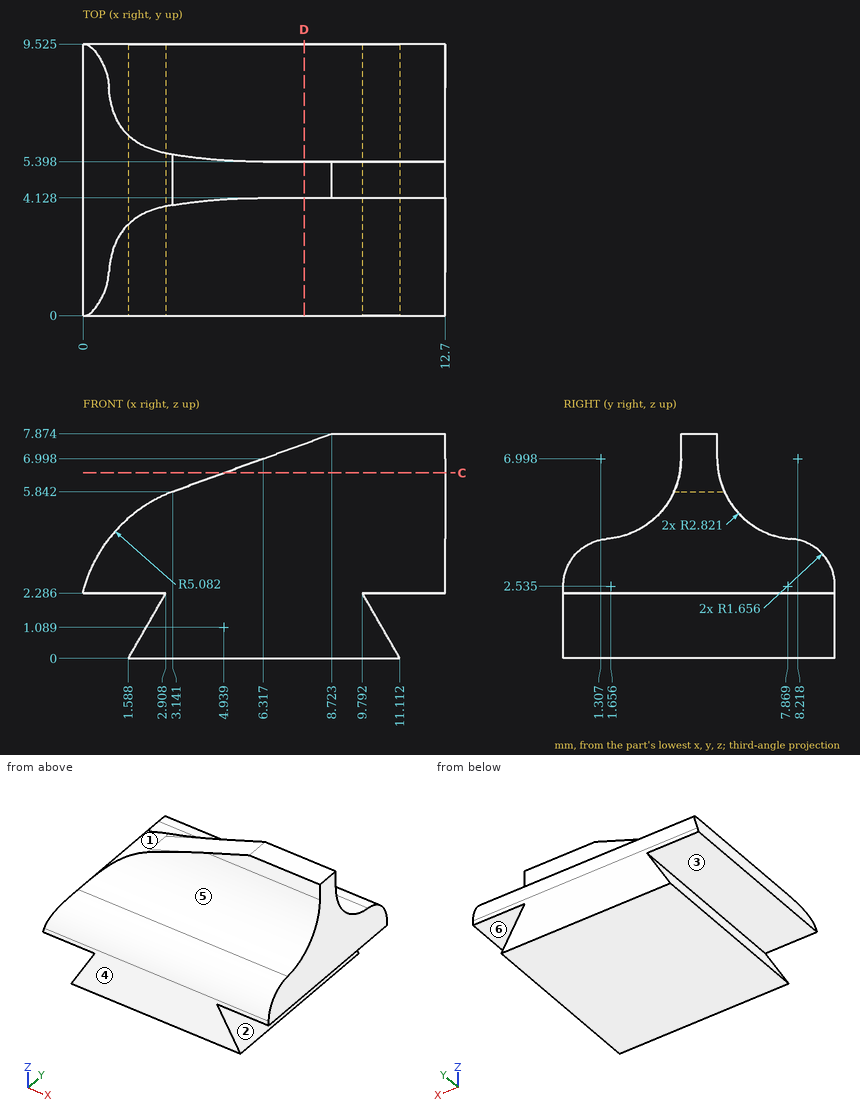
Input: dimensioned drawing with shaded views. Units: mm. Origin: part minimum x, y, z. A direction names the side the tool comes from. Give positions to 0.01 mm unless a question says otherwise; leave off trailing zeros. Loops run counter-clockwise (first coordinate to the right, second up) from the corner with the lowest first, then second, coordinate; pieces in that order, holes last. Notation, with made-up numbers: (46.5, 41) -> (103.5, 41) arc R18 ccw to (103.5, 52) -> close; hole circle Ø11 at (-31.5, -18). An arc over 180 degrees is marked (long way). Return JSON: item names as keys, results as strings.
Item 1: Mould query, pull axis Z, two halves, no side actions, for the marked faces 4, 5 and 6. Classes: released by +Z, released by -Z, zero draft, split by the parting line, or undercut.
Filled in:
{"face 4": "zero draft", "face 5": "released by +Z", "face 6": "undercut"}
Item 2: Pin query (flat end, axial travel): P1, Ø0.9, axis at x = 11, y = 6, coming from the -Z side; P2, Ø1.5, axis at x = 7, y = 1.5, coming from the +Z side; P3, Ø1.5, axis at x = 2.5, y = 5, coming from the +Z side. Return the tip coordinate at first contact, or that it passes through.
Filled in:
{"P1": "z = 0", "P2": "z = 4.34", "P3": "z = 5.88"}
Item 3: Access query for the marked faces 1, 2 and 3. Directions: +Z, -Z, +X, -X, +Y, -Y. A direction counts if a zero-diameter tool reaches every point of the face in a straight line with its end or side. Return the directions, or none.
Filled in:
{"face 1": "+Z, -X, +Y, -Y", "face 2": "+X, +Y, -Y", "face 3": "-X, +Y, -Y"}
Item 4: Section D-D, the plane x = 7.75. Output: boundary loops of the cut face in (y, z) (1 decimal).
Filled in:
{"outline": "(0, 0) -> (9.5, 0) -> (9.5, 2.5) arc R1.7 ccw to (8, 4.2) arc R2.8 cw to (5.4, 7) -> (5.4, 7.5) -> (4.1, 7.5) -> (4.1, 7) arc R2.8 cw to (1.5, 4.2) arc R1.7 ccw to (0, 2.5) -> close"}
Item 5: Line query: line 1 (Z direction, x = 6.5, y = 8) (1 decimal); line 2 (Y direction, x = 8.75, z = 7.5); line 3 (X direction, y = 6.25, z = 1.75). Output: solid intervals per line, ascending.
Filled in:
{"line 1": "0 to 4.2", "line 2": "4.13 to 5.4", "line 3": "2.6 to 10.1"}
Item 6: Section C-C, the plane z = 6.5. Output: boundary loops of the cut face in (x, y).
Filled in:
{"outline": "(4.95, 4.08) -> (12.7, 4.08) -> (12.7, 5.44) -> (4.95, 5.44) -> close"}
